```python
from build123d import *

# Parameters (mm, degrees)
ESBO_O1_R                = 4
RESSALTO_EXTRUS_O1_DEPTH = 11
ESBO_O3_R                = 7.5
RESSALTO_EXTRUS_O3_DEPTH = 3
ESBO_O6_R                = 2.5
CORTE_EXTRUS_O1_DEPTH    = 18.56416807


with BuildPart() as part:
    # Esboço1 → Ressalto-extrusão1 (new body)
    with BuildSketch(Plane(origin=(0, 0, 0), x_dir=(1, 0, 0), z_dir=(0, 1, 0))):
        with Locations(Location((0, 0, 0), (0, 0, 270))):
            Circle(ESBO_O1_R)
    extrude(amount=RESSALTO_EXTRUS_O1_DEPTH)

    # Esboço3 → Ressalto-extrusão3 (add)
    with BuildSketch(Plane.XZ):
        with Locations(Location((0, 0, 0), (0, 0, 270))):
            Circle(ESBO_O3_R)
    extrude(amount=RESSALTO_EXTRUS_O3_DEPTH)

    # Esboço6 → Corte-extrusão1 (cut, through all)
    with BuildSketch(Plane(origin=(0, 11, 0), x_dir=(1, 0, 0), z_dir=(0, 1, 0))):
        with Locations(Location((0, 0, 0), (0, 0, 270))):
            Circle(ESBO_O6_R)
    extrude(amount=-CORTE_EXTRUS_O1_DEPTH, mode=Mode.SUBTRACT)


solid = part.part
```
Build history of the part. All positions in model axes, mm. Coordinates: 2 decimals unless noted, no trailing zeros. Order: outer loops, then holes, each group sorted by start corner. A loop starts at its lowest first (then second) coordinate and runs counter-clockwise, first axis right, second up. Notation, with made-up numbers: (31.5, 11) -> (61.5, 11) arc R7 ccw to (61.5, 17) -> close; hole circle Ø6 at (-3.5, 29). An arc over 180 degrees is marked (long way). Answer in a Markdown table with one row per item. Add a question column.
Q1. Wall check: line 1 along X through (y, z) = (0.5, 0); line 2 along Y through (x, z) = (-5.25, -4.25); line 3 along Z through (x, y) = (0.25, -0.75). Give the ranges that are in metal, low to high. Write a range as [from, to].
Q2. Band-saw the part on C-C, the plane y = 1. List the corners of the cut face in (x, z).
Q3. Band-saw the part on D-D, the plane x = 3. List the corners of the cut face in (y, z), then the cut area to 4 significant figures.
Q4. Mould opens along X. For faces 1 (the face through (-2.44, 4.1, -0.54)), 2 (the face through (-3.905, 5.423, -0.867)), 3 (the face through (-3, 0, -3)) say: +X half, -X half, draft (parallel to the pull), parting line (faces both ways), or undercut.
Q5. Drop flat-ended pins along their axis: pin 1 (3 mm diameter, centred on x = -5, y = 6.5, fed in from -Z); pin 2 (8 mm diameter, centred on x = 0, z = 0, fed in from +Y); pin 3 (1.5 mm diameter, centred on x = 2.5, y = 7.5, fed in from -Z); pin 4 (1.5 mm diameter, centred on y = -0.5, z = -5.5, fed in from +X). Give the stop position or say it passes through.
Q6. Band-saw the part on A-A, the plane x = 0. List the corners of the cut face in (y, z), then the cut area to 3 significant figures.
Q7. Band-saw the part on B-B, the plane z = 0. List the corners of the cut face in (x, y), then the cut area to 3 significant figures.
Answers follow:
| question | item | result |
|---|---|---|
| 1 | line 1 | [-4, -2.5], [2.5, 4] |
| 1 | line 2 | [-3, 0] |
| 1 | line 3 | [-7.5, -2.49], [2.49, 7.5] |
| 2 | outline | circle Ø8 at (0, 0); hole circle Ø5 at (0, 0) |
| 3 | outline | (-3, -6.87) -> (0, -6.87) -> (0, -2.65) -> (11, -2.65) -> (11, 2.65) -> (0, 2.65) -> (0, 6.87) -> (-3, 6.87) -> close |
| 3 | area | 99.45 mm^2 |
| 4 | face 1 | undercut |
| 4 | face 2 | parting line |
| 4 | face 3 | draft |
| 5 | pin 1 | z = -1.94 |
| 5 | pin 2 | y = 11 |
| 5 | pin 3 | z = -3.6 |
| 5 | pin 4 | x = 5.8 |
| 6 | outline | (-3, -7.5) -> (0, -7.5) -> (0, -4) -> (11, -4) -> (11, -2.5) -> (-3, -2.5) -> close; (-3, 2.5) -> (11, 2.5) -> (11, 4) -> (0, 4) -> (0, 7.5) -> (-3, 7.5) -> close |
| 6 | area | 63.0 mm^2 |
| 7 | outline | (-7.5, -3) -> (-2.5, -3) -> (-2.5, 11) -> (-4, 11) -> (-4, 0) -> (-7.5, 0) -> close; (2.5, -3) -> (7.5, -3) -> (7.5, 0) -> (4, 0) -> (4, 11) -> (2.5, 11) -> close |
| 7 | area | 63.0 mm^2 |
